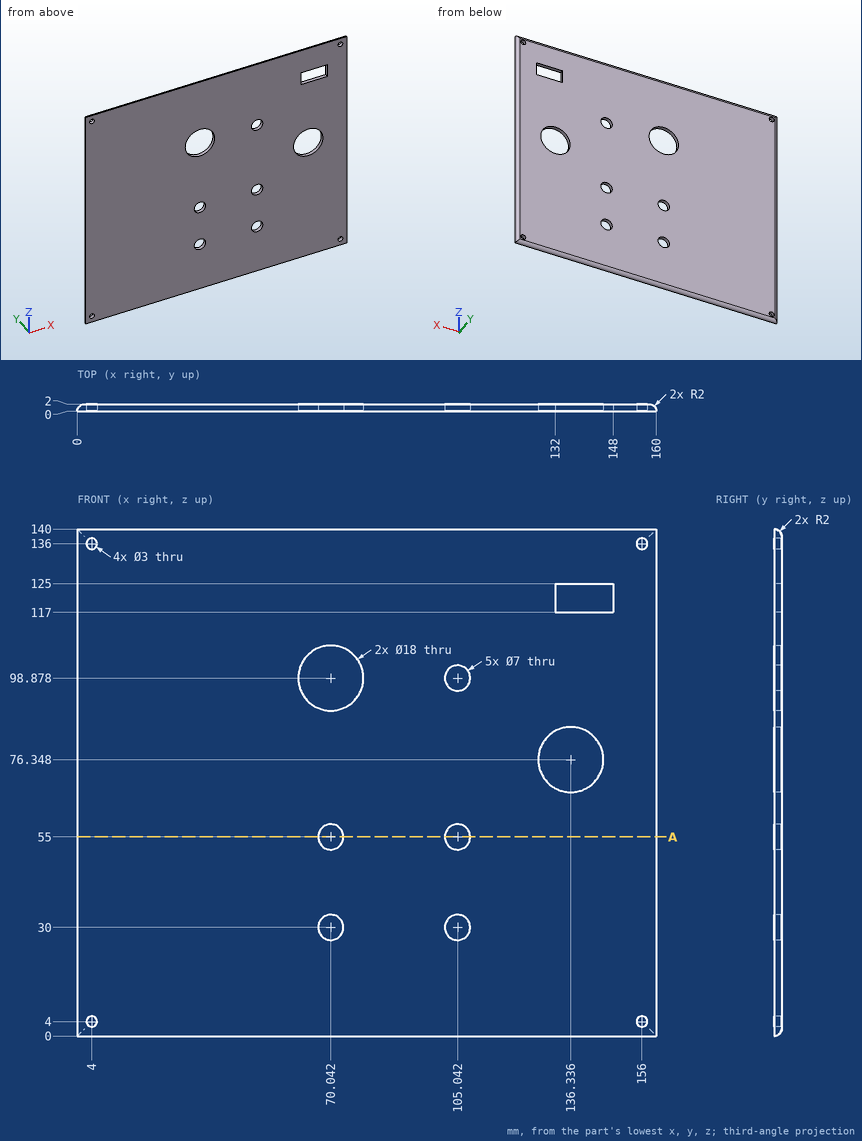
The figure shows three views and two pictorial views of one solid part (mm, origin at its lowest corner). Answer the questions. Give positions to 0.01 mm unless a question says otherwise; leave off trailing zeros. Return JSON: item names as keys, results as strings.
1) Straight lines are drawn through the part: line 1 along X through (y, z) = (0.4, 30); line 2 along Z through (x, y) = (106, 0.2); line 3 along X through (y, z) = (0.2, 75.5). For each, find the intervals that lie inside material, in ascending order. Write a range as [from, to].
Resolved:
{"line 1": "[0.04, 66.54], [73.54, 101.54], [108.54, 159.96]", "line 2": "[0.01, 26.63], [33.37, 51.63], [58.37, 95.51], [102.24, 139.99]", "line 3": "[0.01, 127.38], [145.3, 159.99]"}
2) Each of these flat-tipped pins is pushed along its axis until it touches: pin 1 (1 mm diameter, centred on x = 32.5, y = 1.5, fed in from -Z); pin 2 (1.8 mm diameter, centred on x = 4, z = 4, fed in from -Y); pin 3 (1 mm diameter, centred on x = 140.5, y = 1.5, fed in from +Z); pin 4 (1 mm diameter, centred on y = 1.5, z = 120.5, fed in from -X). Where does it stop, or does it pass through?
Resolved:
{"pin 1": "z = 0.27", "pin 2": "through", "pin 3": "z = 139.73", "pin 4": "x = 0.27"}
3) Section A-A, the plane z = 55 is taken. Give the number of separate pieces and of enclosed holes in the cut face, plus the area to 3 significant figures.
Resolved:
{"separate pieces": "3", "enclosed holes": "0", "area": "290 mm^2"}
